Read the model definition and answer for the solid it produces. Units are mm, in the model's axes. A direction names the side the tool comes from. Coordinates: 2 decimals unless noted, no trailing zeros. Order: outer loops, then holes, each group sorted by start corner. A loop starts at its lowest first (then second) coordinate and runs counter-clockwise, first axis right, second up. Notation, with made-up numbers: (64.25, 31) - (97.25, 31) arc R23 cw to (97.25, 49) - close; hole circle Ø9 at (52.25, 63). An arc over 180 degrees is marked (long way). Write item = value, one per line.
from build123d import *

# Parameters (mm, degrees)
PAD_DEPTH       = 6.5
POCKET_DEPTH    = 6
SKETCH002_R     = 13.5
POCKET001_DEPTH = 1
SKETCH003_W     = 5.4
SKETCH003_H     = 6.5
PAD001_DEPTH    = 4.5
SKETCH010_W     = 3.95
SKETCH010_H     = 6.5
PAD002_DEPTH    = 4.5
SKETCH014_R     = 20.45
SKETCH014_R_2   = 19.5
POCKET008_DEPTH = 0.3
SKETCH015_R     = 2.2
SKETCH015_R_2   = 0.975
PAD003_DEPTH    = 2
POCKET009_DEPTH = 4
POCKET010_DEPTH = 4


with BuildPart() as part:
    # Sketch → Pad (new body)
    with BuildSketch(Plane.XY):
        with BuildLine():
            Line((-22.5019915649, 16), (-22.5019915649, -16))
            Line((-22.5019915649, -16), (-16.2858834577, -17.9000000001))
            ThreePointArc((-16.2858834577, -17.9000000001), (0.2206895737, -24.1989937004), (16.6096357576, -17.5999999999))
            Line((16.6096357576, -17.5999999999), (24.9082802252, -17.45))
            Line((24.9082802252, 17.45), (24.9082802252, -17.45))
            Line((16.6096357576, 17.6), (24.9082802252, 17.45))
            ThreePointArc((16.6096357576, 17.6), (0.2206895736, 24.1989937004), (-16.2858834578, 17.9))
            Line((-22.5019915649, 16), (-16.2858834578, 17.9))
        make_face()
    extrude(amount=PAD_DEPTH)

    # Sketch001 → Pocket (cut)
    with BuildSketch(Plane.XY):
        with BuildLine():
            Line((-14.8539557021, 16.9), (-21.2122180433, 15.55))
            Line((-21.2122180433, 15.55), (-21.2122180433, -15.55))
            Line((-21.2122180433, -15.55), (-14.8539557021, -16.9))
            ThreePointArc((-14.8539557021, -16.9), (-0.0760301383, -22.4998715423), (14.739402973, -17))
            Line((14.739402973, -17), (23.6191552218, -16.4))
            Line((23.6191552218, 16.4), (23.6191552218, -16.4))
            Line((14.739402973, 17), (23.6191552218, 16.4))
            ThreePointArc((14.739402973, 17), (-0.0760301383, 22.4998715423), (-14.8539557021, 16.9))
        make_face()
    extrude(amount=POCKET_DEPTH, mode=Mode.SUBTRACT)

    # Sketch002 (on Face19 of Pocket) → Pocket001 (cut)
    with BuildSketch(Plane(origin=(0, 0, 6), x_dir=(1, 0, 0), z_dir=(0, 0, -1))):
        Circle(SKETCH002_R)
    extrude(amount=-POCKET001_DEPTH, mode=Mode.SUBTRACT)

    # Sketch003 (on Face7 of Pad) → Pad001 (join)
    with BuildSketch(Plane.YZ.offset(24.9082802252)):
        with Locations((-14.75, 3.25)):
            Rectangle(SKETCH003_W, SKETCH003_H)
        with Locations((14.75, 3.25)):
            Rectangle(SKETCH003_W, SKETCH003_H)
    extrude(amount=PAD001_DEPTH)

    # Sketch010 (on Face3 of Pad) → Pad002 (join)
    with BuildSketch(Plane(origin=(-22.5019915649, 0, 0), x_dir=(0, -1, 0), z_dir=(-1, 0, 0))):
        with Locations((-14.025, 3.25)):
            Rectangle(SKETCH010_W, SKETCH010_H)
        with Locations((14.025, 3.25)):
            Rectangle(SKETCH010_W, SKETCH010_H)
    extrude(amount=PAD002_DEPTH)

    # Sketch014 (on Face10 of Pad) → Pocket008 (cut)
    with BuildSketch(Plane.XY.offset(6.5)):
        Circle(SKETCH014_R)
        Circle(SKETCH014_R_2, mode=Mode.SUBTRACT)
    extrude(amount=-POCKET008_DEPTH, mode=Mode.SUBTRACT)

    # Sketch015 (on Face19 of Pocket) → Pad003 (join)
    with BuildSketch(Plane(origin=(0, 0, 6), x_dir=(1, 0, 0), z_dir=(0, 0, -1))):
        with Locations((-18.42, 13.32)):
            Circle(SKETCH015_R)
        with Locations((-18.42, 13.32)):
            Circle(SKETCH015_R_2, mode=Mode.SUBTRACT)
        with Locations((7.27, 18.56)):
            Circle(SKETCH015_R)
        with Locations((7.27, 18.56)):
            Circle(SKETCH015_R_2, mode=Mode.SUBTRACT)
        with Locations((5.37, -19.79)):
            Circle(SKETCH015_R)
        with Locations((5.37, -19.79)):
            Circle(SKETCH015_R_2, mode=Mode.SUBTRACT)
        with Locations((-18.42, -13.32)):
            Circle(SKETCH015_R)
        with Locations((-18.42, -13.32)):
            Circle(SKETCH015_R_2, mode=Mode.SUBTRACT)
    extrude(amount=PAD003_DEPTH)

    # Sketch016 → Pocket009 (cut)
    with BuildSketch(Plane(origin=(0, 0, 0), x_dir=(-1, 0, 0), z_dir=(0, 0, 1))):
        with BuildLine():
            Line((-5, 23.6778377391), (-5, 21.9374109685))
            ThreePointArc((5, 21.9374109685), (0, 22.5), (-5, 21.9374109685))
            Line((5, 23.6778377391), (5, 21.9374109685))
            ThreePointArc((5, 23.6778377391), (0, 24.2), (-5, 23.6778377391))
        make_face()
    extrude(amount=POCKET009_DEPTH, mode=Mode.SUBTRACT)

    # Sketch017 → Pocket010 (cut)
    with BuildSketch(Plane(origin=(0, 0, 0), x_dir=(-1, 0, 0), z_dir=(0, 0, 1))):
        with BuildLine():
            Line((-3.499984119, -22.2261132717), (-3.5, -23.9455632634))
            ThreePointArc((-3.5, -23.9455632634), (0, -24.2000019575), (3.5, -23.9455632634))
            Line((3.5000158811, -22.2261082701), (3.5, -23.9455632634))
            ThreePointArc((-3.499984119, -22.2261132717), (1.60767e-05, -22.5), (3.5000158811, -22.2261082701))
        make_face()
        with BuildLine():
            ThreePointArc((-13.9498796389, -17.6536358312), (-11.25, -19.4855715851), (-8.3135572795, -20.9077680626))
            Line((-8.3135572795, -20.9077680626), (-8.9416927184, -22.487466094))
            ThreePointArc((-15.0038705449, -18.987466094), (-12.1, -20.9578147716), (-8.9416927184, -22.487466094))
            Line((-13.9498796389, -17.6536358312), (-15.0038705449, -18.987466094))
        make_face()
        with BuildLine():
            ThreePointArc((8.3135572795, -20.9077680626), (11.25, -19.4855715851), (13.9498796389, -17.6536358312))
            Line((13.9498796389, -17.6536358312), (15.0038705449, -18.987466094))
            ThreePointArc((8.9416927184, -22.487466094), (12.1, -20.9578147716), (15.0038705449, -18.987466094))
            Line((8.3135572795, -20.9077680626), (8.9416927184, -22.487466094))
        make_face()
    extrude(amount=POCKET010_DEPTH, mode=Mode.SUBTRACT)


solid = part.part
1) Determine the mould class of faces 6 (the face through (27, -17.45, 3)), 7 (the face through (-20.618, 13.223, 5.014)), 8 (the face through (-27.002, -14, 3)) for opening direction X: pulls with the +X half, pulls with the -X half, needs draft (parallel to the pull), parting line crosses it, or undercut.
Returned:
face_6 = needs draft
face_7 = undercut
face_8 = pulls with the -X half
2) The part is cut by section D-D (z = 2.75). Count the separate pieces of the cut face and the enclosed holes in it, and give its area (3 significant figures).
Returned:
separate_pieces = 4
enclosed_holes = 0
area = 262 mm^2
3) For faces 1 (the face through (0.474, 24.195, 4.649)), 2 (the face through (-19.437, -16.937, 3.204)), 3 (the face through (-5, -23, 2)), 4 (the face through (-14.47, 18.31, 1.97)), 5 (the face through (-17, 14, 4)), determine the directions among +Z, -Z, +X, -X, +Y, -Y from which every point of the face is accessible in a straight line to the end or side of a thin tool.
Returned:
face_1 = +Z, -Z, +Y
face_2 = +Z, -Z, -X, -Y
face_3 = -Z, -Y
face_4 = -Z, +Y
face_5 = -Z
4) The part is cut by section B-B (x = 0). Determine the outline of the cut face in (y, z).
Returned:
outline = (-24.2, 4) - (-22.5, 4) - (-22.5, 6) - (-13.5, 6) - (-13.5, 6.5) - (-19.5, 6.5) - (-19.5, 6.2) - (-20.45, 6.2) - (-20.45, 6.5) - (-24.2, 6.5) - close; (13.5, 6) - (22.5, 6) - (22.5, 4) - (24.2, 4) - (24.2, 6.5) - (20.45, 6.5) - (20.45, 6.2) - (19.5, 6.2) - (19.5, 6.5) - (13.5, 6.5) - close
5) The part is cut by section C-C (y = -18.56). Determine the outline of the cut face in (x, z) (3 decimals), and give its area (3 significant figures).
Returned:
outline = (-15.53, 0) - (-12.719, 0) - (-12.719, 6) - (5.07, 6) - (5.07, 4) - (6.295, 4) - (6.295, 6) - (8.245, 6) - (8.245, 4) - (9.47, 4) - (9.47, 6) - (12.719, 6) - (12.719, 0) - (15.53, 0) - (15.53, 6.5) - (8.587, 6.5) - (8.587, 6.2) - (5.981, 6.2) - (5.981, 6.5) - (-5.981, 6.5) - (-5.981, 6.2) - (-8.587, 6.2) - (-8.587, 6.5) - (-15.53, 6.5) - close
area = 52.6 mm^2
6) Flat-ended cylindrical pins translate along their axes: pin 1 Ø2 at (x, y) = (8, -18) entering from -Z; pin 2 Ø3 at (y, z) = (5.5, 2.5) entering from -X; pin 3 Ø3 at (x, z) = (-15, 3) entering from +Y; pin 4 Ø16 at (x, y) = (0, 0) entering from -Z. Find the tip coordinate at first contact, or state that the pin passes through.
Returned:
pin_1 = 4
pin_2 = -22.5
pin_3 = 19.82
pin_4 = through
7) The part is cut by section A-A (y = 0). Determine the outline of the cut face in (x, z).
Returned:
outline = (-22.5, 0) - (-21.21, 0) - (-21.21, 6) - (-13.5, 6) - (-13.5, 6.5) - (-19.5, 6.5) - (-19.5, 6.2) - (-20.45, 6.2) - (-20.45, 6.5) - (-22.5, 6.5) - close; (13.5, 6) - (23.62, 6) - (23.62, 0) - (24.91, 0) - (24.91, 6.5) - (20.45, 6.5) - (20.45, 6.2) - (19.5, 6.2) - (19.5, 6.5) - (13.5, 6.5) - close
8) Straight lines are drawn through the part: line 1 along X through (y, z) = (-13.32, 4.9) (3 decimals); line 2 along X through (y, z) = (4.5, 2.5); line 3 along Y through (x, z) = (0, 6.4). For each, find the intervals that lie inside material, in ascending order. Write a range as from..to.
Returned:
line_1 = -27.002..-21.212, -20.62..-19.395, -17.445..-16.22, 23.619..29.408
line_2 = -22.5..-21.21, 23.62..24.91
line_3 = -24.2..-20.45, -19.5..-13.5, 13.5..19.5, 20.45..24.2
